Geometry: final body of the model. Coordinates: model frame, mm. Face numbers are marked on the shaded views. Give positions to 0.01 mm unless a question says otherwise; leave off trailing zeros. Write each loop counter-clockwise with the first axis right and the second up, starting at its lowest first coordinate (ties: lowest second). Pieces come first, ordered by that corner, then holes. Notation, with made-up numbers: (-25.75, 89.25) -> (-10.75, 89.25) arc R36 cw to (-10.75, 127.25) -> close; hole circle Ø7 at (1, 25.5). An arc over 180 degrees is marked (long way). Use CSV: the item, a comma, the result in double quotes. Start each with the question number.
1) Section D-D (z = 0). Output: boundary loops of the cut face in (x, y), plus the area to 4 significant figures.
2) Material intervals for line 1 (X direction, y = 5.2, z = 0); line 2 (X direction, y = 4.9, z = 23.55); line 3 (Z direction, x = 0, y = 6.6), sorted ascending. Write a range as [from, to].
3) Section A-A (x = 0). Output: boundary loops of the cut face in (y, z), plus the area to 3 significant figures.
4) Section C-C (z = -23.55). Output: boundary loops of the cut face in (x, y).
5) Draft query along X for the marked faces 1 and 2. Return one class per face: pulls with the +X half, pulls with the -X half, needs draft (parallel to the pull), parting line crosses it, or undercut.
6) Section B-B (x = -34). Output: boundary loops of the cut face in (y, z), plus the area to 3 significant figures.
7) Contact query for flat-ended pins moving along their axis: P1, Ø2.5, axis at y = 7, z = -42, coming from the -X side; P2, Ø2.5, axis at x = 33.5, y = 6.5, coming from the +Z side; P3, Ø10, axis at x = -12, z = 4, coming from the -Y side; P4, Ø3, axis at x = -8, z = -43.5, coming from the +Y side. Output: stop coordinate, or through.
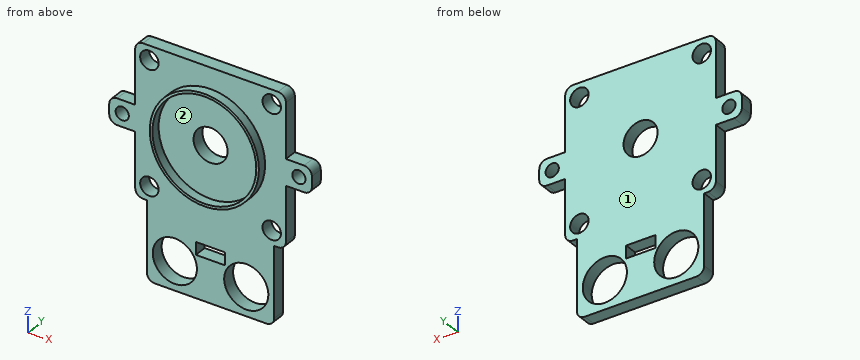
```python
from build123d import *

# Parameters (mm, degrees)
SKETCH1_R           = 21
SKETCH1_R_2         = 20
BOSS_EXTRUDE1_DEPTH = 3.5
SKETCH2_R           = 3.55
SKETCH2_R_2         = 6.55
SKETCH2_R_3         = 2.55
SKETCH2_R_4         = 8.5
SKETCH2_W           = 11.2
SKETCH2_H           = 4.84
BOSS_EXTRUDE2_DEPTH = 5
SKETCH3_W           = 11.2
SKETCH3_H           = 4.84
SKETCH3_W_2         = 49
SKETCH3_H_2         = 8
SKETCH3_R           = 8.5
IGNORE_DEPTH        = 5
SKETCH4_R           = 8.5
SKETCH4_W           = 11.2
SKETCH4_H           = 4.84
CUT_EXTRUDE2_DEPTH  = 6
FILLET1_R           = 3


with BuildPart() as part:
    # Sketch1 → Boss-Extrude1 (new body)
    with BuildSketch(Plane(origin=(0, 0, 0), x_dir=(1, 0, 0), z_dir=(0, 1, 0))):
        Circle(SKETCH1_R)
        Circle(SKETCH1_R_2, mode=Mode.SUBTRACT)
    extrude(amount=BOSS_EXTRUDE1_DEPTH)

    # Sketch2 → Boss-Extrude2 (add)
    with BuildSketch(Plane(origin=(0, 3.5, 0), x_dir=(1, 0, 0), z_dir=(0, 1, 0))):
        Polygon((-29, -5), (-29, -29), (29, -29), (29, -5), (39, -5), (39, 5), (29, 5), (29, 29), (24.5, 29), (24.5, 51), (-24.5, 51), (-24.5, 29), (-29, 29), (-29, 5), (-39, 5), (-39, -5), align=None)
        with Locations((-23.55, -23.55)):
            Circle(SKETCH2_R, mode=Mode.SUBTRACT)
        with Locations((23.55, -23.55)):
            Circle(SKETCH2_R, mode=Mode.SUBTRACT)
        Circle(SKETCH2_R_2, mode=Mode.SUBTRACT)
        with Locations((-23.55, 23.55)):
            Circle(SKETCH2_R, mode=Mode.SUBTRACT)
        with Locations((23.55, 23.55)):
            Circle(SKETCH2_R, mode=Mode.SUBTRACT)
        with Locations((-34, 0)):
            Circle(SKETCH2_R_3, mode=Mode.SUBTRACT)
        with Locations((34, 0)):
            Circle(SKETCH2_R_3, mode=Mode.SUBTRACT)
        with Locations((13.76, 39)):
            Circle(SKETCH2_R_4, mode=Mode.SUBTRACT)
        with Locations((-13.76, 39)):
            Circle(SKETCH2_R_4, mode=Mode.SUBTRACT)
        with Locations((0, 46.28)):
            Rectangle(SKETCH2_W, SKETCH2_H, mode=Mode.SUBTRACT)
    extrude(amount=BOSS_EXTRUDE2_DEPTH)

    # Sketch3 → Ignore (add)
    with BuildSketch(Plane(origin=(0, 3.5, 0), x_dir=(1, 0, 0), z_dir=(0, 1, 0))):
        with Locations((0, 46.28)):
            Rectangle(SKETCH3_W, SKETCH3_H)
        with Locations((0, 55)):
            Rectangle(SKETCH3_W_2, SKETCH3_H_2)
        with Locations((13.76, 39)):
            Circle(SKETCH3_R)
        with Locations((-13.76, 39)):
            Circle(SKETCH3_R)
    extrude(amount=IGNORE_DEPTH)

    # Sketch4 → Cut-Extrude2 (cut, through all)
    with BuildSketch(Plane(origin=(0, 3.5, 0), x_dir=(1, 0, 0), z_dir=(0, 1, 0))):
        with Locations((-13.75, 48)):
            Circle(SKETCH4_R)
        with Locations((13.75, 48)):
            Circle(SKETCH4_R)
        with Locations((-0.079148889, 40.42)):
            Rectangle(SKETCH4_W, SKETCH4_H)
    extrude(amount=CUT_EXTRUDE2_DEPTH, mode=Mode.SUBTRACT)

    # Fillet1
    fillet1_edges = [part.edges().sort_by_distance(p)[0] for p in [
        (-29, 6, 29),
        (29, 6, 29),
        (39, 6, 5),
        (39, 6, -5),
        (29, 6, -29),
        (-29, 6, -29),
        (-39, 6, -5),
        (-39, 6, 5),
        (24.5, 6, -59),
        (-24.5, 6, -59),
    ]]
    fillet(fillet1_edges, radius=FILLET1_R)


solid = part.part
```
Answers follow:
1,outline,"(-39, 3.5) -> (-36.55, 3.5) -> (-36.55, 8.5) -> (-39, 8.5) -> close; (-31.45, 3.5) -> (-21, 3.5) -> (-21, 0) -> (-20, 0) -> (-20, 3.5) -> (-6.55, 3.5) -> (-6.55, 8.5) -> (-31.45, 8.5) -> close; (6.55, 3.5) -> (20, 3.5) -> (20, 0) -> (21, 0) -> (21, 3.5) -> (31.45, 3.5) -> (31.45, 8.5) -> (6.55, 8.5) -> close; (36.55, 3.5) -> (39, 3.5) -> (39, 8.5) -> (36.55, 8.5) -> close"
1,area,"280.5 mm^2"
2,line 1,"x = [-39, -36.55], [-31.45, -6.55], [6.55, 31.45], [36.55, 39]"
2,line 2,"x = [-29, -27.1], [-20, 20], [27.1, 29]"
2,line 3,"z = [-59, -42.84], [-38, -6.55], [6.55, 29]"
3,outline,"(0, -21) -> (3.5, -21) -> (3.5, -38) -> (8.5, -38) -> (8.5, -6.55) -> (3.5, -6.55) -> (3.5, -20) -> (0, -20) -> close; (0, 20) -> (3.5, 20) -> (3.5, 6.55) -> (8.5, 6.55) -> (8.5, 29) -> (3.5, 29) -> (3.5, 21) -> (0, 21) -> close; (3.5, -59) -> (8.5, -59) -> (8.5, -42.84) -> (3.5, -42.84) -> close"
3,area,"357 mm^2"
4,outline,"(-29, 3.5) -> (-27.1, 3.5) -> (-27.1, 8.5) -> (-29, 8.5) -> close; (-20, 3.5) -> (20, 3.5) -> (20, 8.5) -> (-20, 8.5) -> close; (27.1, 3.5) -> (29, 3.5) -> (29, 8.5) -> (27.1, 8.5) -> close"
5,face 1,"needs draft"
5,face 2,"undercut"
6,outline,"(3.5, -5) -> (8.5, -5) -> (8.5, -2.55) -> (3.5, -2.55) -> close; (3.5, 2.55) -> (8.5, 2.55) -> (8.5, 5) -> (3.5, 5) -> close"
6,area,"24.5 mm^2"
7,P1,"stops at x = -24.5"
7,P2,"stops at z = 5"
7,P3,"stops at y = 3.5"
7,P4,"stops at y = 8.5"
